Here's how the part is built. I have some questions about the finished solid (model axes, mm). A direction names the side the tool comes from. Coordinates: 2 decimals unless noted, no trailing zeros. Write each loop counter-clockwise with the first axis right and the second up, starting at its lowest first coordinate (ties: lowest second). Pieces come first, ordered by that corner, then holes. Notation, with made-up numbers: (5.5, -15) -> (47.5, -15) arc R29 ccw to (47.5, 6) -> close; hole circle Ø1 at (78, 83.5). An arc over 180 degrees is marked (long way). Use a Markdown table: item, result. Add a question column.
```python
from build123d import *

# Parameters (mm, degrees)
IZIM1_R                     = 1.5
Y_KSEKLIK_EKSTR_ZYON1_DEPTH = 1.6


with BuildPart() as part:
    # Çizim1 → Yükseklik-Ekstrüzyon1 (new body)
    with BuildSketch(Plane.XY):
        Polygon((0, -55), (-10, -45), (-10, 45), (10, 45), (90, 45), (90, -45), (80, -55), (70, -45), (70, 32), (50, 32), (50, -45), (40, -55), (30, -45), (30, 32), (10, 32), (10, -45), align=None)
        with Locations((-7, 29)):
            Circle(IZIM1_R, mode=Mode.SUBTRACT)
        with Locations((7, 29)):
            Circle(IZIM1_R, mode=Mode.SUBTRACT)
        with Locations((33, 29)):
            Circle(IZIM1_R, mode=Mode.SUBTRACT)
        with Locations((47, 29)):
            Circle(IZIM1_R, mode=Mode.SUBTRACT)
        with Locations((73, 29)):
            Circle(IZIM1_R, mode=Mode.SUBTRACT)
        with Locations((87, 29)):
            Circle(IZIM1_R, mode=Mode.SUBTRACT)
    extrude(amount=Y_KSEKLIK_EKSTR_ZYON1_DEPTH)


solid = part.part
```
Q1. Suppose I cut it at C-C, the plane z = 0.5. Write out the boundary of the cut face in (x, y).
Q2. Please list where these lines run through material, in increasing order: line 1 (X direction, y = -18, z = 0.75); line 2 (Y direction, x = 46.5, z = 0.5); line 3 (Y direction, x = 55, z = 1).
Q3. Will these pins go through, and if not, where does the flat tip stop? pin 1 (5 mm diameter, centred on x = 87, y = 29, fed in from +Z); pin 2 (0.5 mm diameter, centred on x = 56, z = 0.5, fed in from -Y).
Q4. Thinking about a two-plate mould opening in Y: for faces 1 (the flat face through (75, -50, 1)), 2 (the cylindrical face through (-7.195, 30.487, 0.789)), 3 (the flat face through (41, -4, 1.6)), which applies, released by +Y, released by -Y, zero draft, split by the parting line, or undercut?
Q5. Suppose I cut it at D-D, the plane y = -48. Write out the boundary of the cut face in (x, z), and give its area (3 significant figures).
Q6. Suppose I cut it at B-B, the plane y = 26. Write out the boundary of the cut face in (x, z).
Q7. Suppose I cut it at A-A, the plane x = 87. Write out the boundary of the cut face in (y, z), and give its area (3 significant figures).
Q8. Which directions (+Z, -Z, +X, -X, +Y, -Y) give clear straight access to the entire face, cutting with the end or side of a thin tool? Please do faces 4 (the flat face through (85, -50, 1)), 5 (the flat face through (35, -50, 1)).
Answer key:
| question | item | result |
|---|---|---|
| 1 | outline | (-10, -45) -> (0, -55) -> (10, -45) -> (10, 32) -> (30, 32) -> (30, -45) -> (40, -55) -> (50, -45) -> (50, 32) -> (70, 32) -> (70, -45) -> (80, -55) -> (90, -45) -> (90, 45) -> (-10, 45) -> close; hole circle Ø3 at (-7, 29); hole circle Ø3 at (7, 29); hole circle Ø3 at (33, 29); hole circle Ø3 at (47, 29); hole circle Ø3 at (73, 29); hole circle Ø3 at (87, 29) |
| 2 | line 1 | x = -10 to 10, 30 to 50, 70 to 90 |
| 2 | line 2 | y = -48.5 to 27.59, 30.41 to 45 |
| 2 | line 3 | y = 32 to 45 |
| 3 | pin 1 | stops at z = 1.6 |
| 3 | pin 2 | stops at y = 32 |
| 4 | face 1 | released by -Y |
| 4 | face 2 | undercut |
| 4 | face 3 | zero draft |
| 5 | outline | (-7, 0) -> (7, 0) -> (7, 1.6) -> (-7, 1.6) -> close; (33, 0) -> (47, 0) -> (47, 1.6) -> (33, 1.6) -> close; (73, 0) -> (87, 0) -> (87, 1.6) -> (73, 1.6) -> close |
| 5 | area | 67.2 mm^2 |
| 6 | outline | (-10, 0) -> (10, 0) -> (10, 1.6) -> (-10, 1.6) -> close; (30, 0) -> (50, 0) -> (50, 1.6) -> (30, 1.6) -> close; (70, 0) -> (90, 0) -> (90, 1.6) -> (70, 1.6) -> close |
| 7 | outline | (-48, 0) -> (27.5, 0) -> (27.5, 1.6) -> (-48, 1.6) -> close; (30.5, 0) -> (45, 0) -> (45, 1.6) -> (30.5, 1.6) -> close |
| 7 | area | 144 mm^2 |
| 8 | face 4 | +Z, -Z, +X, -Y |
| 8 | face 5 | +Z, -Z, -Y |
